Design review of the part built by this model. Coordinates are the model's own, in mm. A direction names the side the tool comes from. Round coordinates to 2 decimals unless told otherwise and drop trailing zeros. Loops run counter-clockwise (first coordinate to the right, second up) from the corner with the lowest first, then second, coordinate; pieces in that order, holes last. Notation, with made-up numbers: M 89.5,57.25 L 128.5,57.25 A16 ccw 128.5,82.25 Z; hole C 48,68.25 d10. An arc over 180 degrees is marked long. Answer as CSV lines item,"result". Start each with the question number.
from build123d import *

# Parameters (mm, degrees)
SKIZZE1_R                       = 4
AUFSATZ_LINEAR_AUSTRAGEN1_DEPTH = 3


with BuildPart() as part:
    # Skizze1 → Aufsatz-Linear austragen1 (new body)
    with BuildSketch(Plane.XY):
        with BuildLine():
            Line((0, 0), (110, 0))
            Line((110, 0), (110, 7.087121525))
            ThreePointArc((110, 7.087121525), (95, 30), (110, 52.912878475))
            Line((110, 52.912878475), (110, 95))
            Line((110, 95), (0, 95))
            Line((0, 95), (0, 0))
        make_face()
        with Locations((25, 80)):
            Circle(SKIZZE1_R, mode=Mode.SUBTRACT)
        with Locations((55, 80)):
            Circle(SKIZZE1_R, mode=Mode.SUBTRACT)
        with Locations((85, 80)):
            Circle(SKIZZE1_R, mode=Mode.SUBTRACT)
        with BuildLine():
            Line((25, 25), (65, 25))
            ThreePointArc((65, 25), (70, 20), (65, 15))
            Line((65, 15), (25, 15))
            ThreePointArc((25, 15), (20, 20), (25, 25))
        make_face(mode=Mode.SUBTRACT)
    extrude(amount=AUFSATZ_LINEAR_AUSTRAGEN1_DEPTH)


solid = part.part
Item 1: Consider section A-A, the plane y = 80. Write out the cut boundary in (x, z), then the cut area to 3 significant figures.
Item 2: Tool access review of faces 5 (the face through (45, 25, 1)), 6 (the face through (0, 48, 1)): name each direction out of +Z, -Z, +X, -X, +Y, -Y from which nothing blocks a thin tool from reaching the whole face with its end or side.
Item 3: Consider section C-C, the plane x = 85. Write out the cut boundary in (y, z), then the cut area to 3 significant figures.
Item 4: Consider section B-B, the plane x = 55. Write out the cut boundary in (y, z), then the cut area to 3 significant figures.
Item 5: Consider section D-D, the plane z = 0.9. Write out the cut boundary in (x, y).
Item 6: To check wall thickness, follow line 1 (Y direction, x = 25, z = 1.25); line 2 (Y direction, x = 23, z = 1.3); line 3 (Y direction, x = 85, z = 1.5). State the ranges of each line that lie inside material, in increasing order.
Item 7: The part is to be moulded in two halves that separate along Y. For faces 1 (the face through (110, 3, 1)), 2 (the face through (54, 0, 1)), 3 (the face through (95, 30, 1)), 4 (the face through (84.133, 76.095, 1.479)), say which applies: +Y half, -Y half, draft (parallel to the pull), parting line (faces both ways), or undercut.
Item 8: Insertion check: pin 1 Ø1.5 at (y, z) = (32.5, 1) entering from +X. The pin has a flat end and moves straight along its axis. Give the tip position at first contact, or say it passes through.
Found:
1,outline,"M 0,0 L 21,0 L 21,3 L 0,3 Z; M 29,0 L 51,0 L 51,3 L 29,3 Z; M 59,0 L 81,0 L 81,3 L 59,3 Z; M 89,0 L 110,0 L 110,3 L 89,3 Z"
1,area,"258 mm^2"
2,face 5,"+Z, -Z"
2,face 6,"+Z, -Z, -X, +Y, -Y"
3,outline,"M 0,0 L 76,0 L 76,3 L 0,3 Z; M 84,0 L 95,0 L 95,3 L 84,3 Z"
3,area,"261 mm^2"
4,outline,"M 0,0 L 15,0 L 15,3 L 0,3 Z; M 25,0 L 76,0 L 76,3 L 25,3 Z; M 84,0 L 95,0 L 95,3 L 84,3 Z"
4,area,"231 mm^2"
5,outline,"M 0,0 L 110,0 L 110,7.09 A25 cw 110,52.91 L 110,95 L 0,95 Z; hole C 25,80 d8; hole M 25,15 L 65,15 A5 ccw 65,25 L 25,25 A5 ccw Z; hole C 55,80 d8; hole C 85,80 d8"
6,line 1,"y = 0 to 15, 25 to 76, 84 to 95"
6,line 2,"y = 0 to 15.42, 24.58 to 76.54, 83.46 to 95"
6,line 3,"y = 0 to 76, 84 to 95"
7,face 1,"draft"
7,face 2,"-Y half"
7,face 3,"undercut"
7,face 4,"undercut"
8,pin 1,"stops at x = 95.21"
